Build history of the part. All positions in model axes, mm. Face numbers are marked on the shaded views. A direction names the side the tool comes from. Give positions to 0.01 mm unless a question says otherwise; leave off trailing zeros. Write each question's results on one line, items separated by ' | '. Start each with the question number.
1) Tool access for the marked faces 3 and 4: list every direction of +Z, -Z, +X, -X, +Y, -Y with a clear straight run to the whole face (end or side of a thin tool).
2) Drop flat-ended pins along their axis: pin 1 Ø1.3 at (y, z) = (-1, 4.5) entering from +X; pin 2 Ø5 at (y, z) = (-1, 3.5) entering from -X; pin 3 Ø2 at (x, z) = (-3, 8) entering from +Y. Give the stop position or say it passes through.
3) Two-plate mould, pull along X, no slides. Class the marked faces 1 and 2: +X half, -X half, draft (parallel to the pull), parting line (faces both ways), or undercut.
4) Drill centre lines: line 1 along Y through (x, z) = (-1, 12); line 2 along Y through (x, z) = (0.5, 1); line 3 along X through (y, z) = (0.5, 13.25). Where is each one in solid material? Low to high. Write a range as from..to.
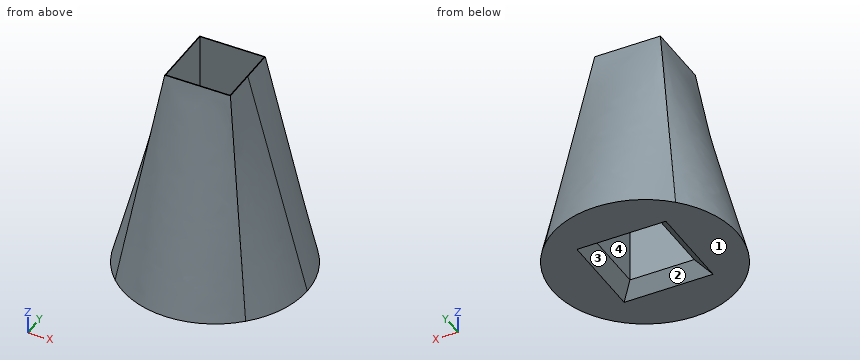
from build123d import *

# Parameters (mm, degrees)
F0_R     = 6
F2_W     = 4.27
F2_H     = 4.27
F4_W     = 4.18
F4_H     = 4.18
F5_DEPTH = 25
F6_SIZE2 = 0.8
F6_SIZE  = 0.8


with BuildPart() as f3:
    # F0 (on Top) → F3 section 0
    with BuildSketch(Plane.XY):
        Circle(F0_R)
    # F2 (on offset) → F3 section 1
    with BuildSketch(Plane.XY.offset(14)):
        Rectangle(F2_W, F2_H)
    loft()

    # F4 (on face) → F5 (cut)
    with BuildSketch(Plane.XY.offset(14)):
        Rectangle(F4_W, F4_H)
    extrude(amount=-F5_DEPTH, mode=Mode.SUBTRACT)

    # F6
    f6_edges = [f3.edges().sort_by_distance(p)[0] for p in [
        (-2.09, 0, 0),
        (0, -2.09, 0),
        (2.09, 0, 0),
        (0, 2.09, 0),
    ]]
    chamfer(f6_edges, length=F6_SIZE, length2=F6_SIZE2)


solid = f3.part
Results:
1) face 3: -Z | face 4: +Z, -Z
2) pin 1: x = 4.88 | pin 2: x = -5.69 | pin 3: y = 3.57
3) face 1: draft | face 2: undercut
4) line 1: -2.64..-2.09, 2.09..2.64 | line 2: -5.7..-2.09, 2.09..5.7 | line 3: -2.34..-2.09, 2.09..2.34
